```python
from build123d import *

# Parameters (mm, degrees)
F0_R     = 52.5
F0_R_2   = 39
F1_DEPTH = 2
F2_R     = 0.25
F3_R     = 1.75
F4_DEPTH = 2.001


with BuildPart() as f1:
    # F0 (on Top) → F1 (new body)
    with BuildSketch(Plane.XY):
        Circle(F0_R)
        Circle(F0_R_2, mode=Mode.SUBTRACT)
    extrude(amount=F1_DEPTH)

    # F2
    f2_edges = [f1.edges().sort_by_distance(p)[0] for p in [
        (-52.5, 0, 2),
        (-39, 0, 2),
    ]]
    fillet(f2_edges, radius=F2_R)

    # F3 (on Top) → F4 (cut, through all)
    with BuildSketch(Plane.XY):
        with Locations((48.5, 0)):
            Circle(F3_R)
        with Locations((0, 48.5)):
            Circle(F3_R)
        with Locations((-48.5, 0)):
            Circle(F3_R)
        with Locations((0, -48.5)):
            Circle(F3_R)
    extrude(amount=F4_DEPTH, mode=Mode.SUBTRACT)


solid = f1.part
```
Could you check a few things on this model? Use its own coordinates, in mm. Round coordinates to 2 decimals unless told otherwise and drop trailing zeros. Loops run counter-clockwise (first coordinate to the right, second up) from the corner with the lowest first, then second, coordinate; pieces in that order, holes last. Notation, with made-up numbers: (62.5, 44.5) - (99.5, 44.5) arc R19 cw to (99.5, 60.5) - close; hole circle Ø1 at (40.25, 59.25). An arc over 180 degrees is marked (long way). Use CSV: the item, a comma, the result in double quotes.
Item 1: If we section it at B-B on z = 0.4: List the corners of the cut face in (x, y) for me, then the cut area to 3 significant figures.
Here are the results:
outline,"circle Ø105 at (0, 0); hole circle Ø3.5 at (-48.5, 0); hole circle Ø78 at (0, 0); hole circle Ø3.5 at (0, -48.5); hole circle Ø3.5 at (0, 48.5); hole circle Ø3.5 at (48.5, 0)"
area,"3,840 mm²"
Item 2: Will these pins go through, and if not, where does the flat tip stop? pin 1 (4.5 mm diameter, centred on x = 48.5, y = 0, fed in from -Z); pin 2 (1 mm diameter, centred on y = 39, z = 1.5, fed in from +X).
Here are the results:
pin 1,"stops at z = 0"
pin 2,"stops at x = 35.69"
Item 3: If we section it at A-A on x = 0: List the corners of the cut face in (y, z) for me.
Here are the results:
outline,"(-52.5, 0) - (-50.25, 0) - (-50.25, 2) - (-52.25, 2) arc R0.25 ccw to (-52.5, 1.75) - close; (-46.75, 0) - (-39, 0) - (-39, 1.75) arc R0.25 ccw to (-39.25, 2) - (-46.75, 2) - close; (39, 0) - (46.75, 0) - (46.75, 2) - (39.25, 2) arc R0.25 ccw to (39, 1.75) - close; (50.25, 0) - (52.5, 0) - (52.5, 1.75) arc R0.25 ccw to (52.25, 2) - (50.25, 2) - close"
Item 4: I need wall thicknesses on L1, parallel to Y at x = 0, z = 0.5; L2, parallel to Y at x = 1.5, z = 1; L3, parallel to X at y = -0.5, z = 0.5. Which ranges of each line are inside material? Lowest first, please. Write a range as [from, to].
Here are the results:
L1,"y = [-52.5, -50.25], [-46.75, -39], [39, 46.75], [50.25, 52.5]"
L2,"y = [-52.48, -49.4], [-47.6, -38.97], [38.97, 47.6], [49.4, 52.48]"
L3,"x = [-52.5, -50.18], [-46.82, -39], [39, 46.82], [50.18, 52.5]"
Item 5: If we mould it in two halves opening along X, with no side actions, what happens to faces 1 (the cylindrical face through (50.076, 15.77, 0.863)), 2 (the cylindrical face through (-5.077, 38.668, 0.863)), 3 (the flat face through (-8, 39, 2))? For each: pulls with the +X half, pulls with the -X half, needs draft (parallel to the pull), parting line crosses it, or undercut.
Here are the results:
face 1,"parting line crosses it"
face 2,"undercut"
face 3,"needs draft"
